The model under review builds one solid part; all positions refer to its coordinate system, in mm. Face numbers are marked on the shaded views. Coordinates: 2 decimals unless noted, no trailing zeros. Order: outer loops, then holes, each group sorted by start corner. A loop starts at its lowest first (then second) coordinate and runs counter-clockwise, first axis right, second up. Notation, with made-up numbers: (47, -4.75) -> (100, -4.75) arc R17 cw to (100, -0.75) -> close; hole circle Ø7 at (79.5, 16). An arc over 180 degrees is marked (long way). Put each result on its own line as item: value.
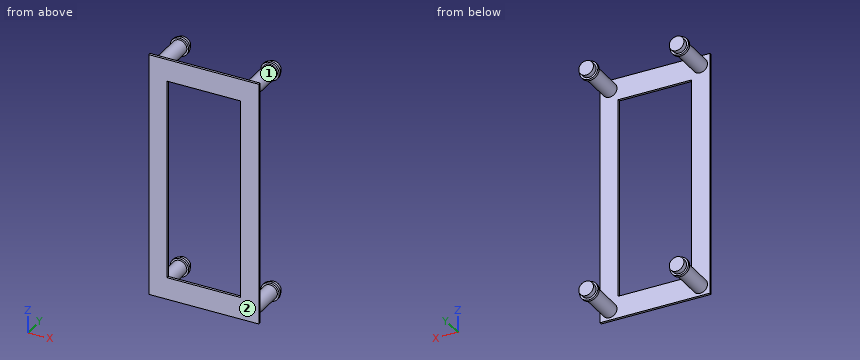
Autodesk Fusion 360 part; units mm, degrees
sketch "Sketch1" plane through (0, 0, 0) normal (0, 1, 0) x (1, 0, 0)
  line L0 (22.5, 50) -> (-22.5, 50)
  line L1 (-22.5, 50) -> (-22.5, -50)
  line L2 (-22.5, -50) -> (22.5, -50)
  line L3 (22.5, -50) -> (22.5, 50)
  line L4 (22.5, 50) -> (-22.5, -50) construction
  line L5 (-22.5, 50) -> (22.5, -50) construction
  line L6 (15, 41) -> (-15, 41)
  line L7 (-15, 41) -> (-15, -41)
  line L8 (-15, -41) -> (15, -41)
  line L9 (15, -41) -> (15, 41)
  line L10 (15, 41) -> (-15, -41) construction
  line L11 (-15, 41) -> (15, -41) construction
  dimension "d1" = 45
  dimension "d2" = 100
  dimension "d3" = 30
  dimension "d4" = 82
extrude "Extrude1" add sketch "Sketch1" along normal blind 1
sketch "Sketch2" plane through (0, 1, 0) normal (0, 1, 0) x (-1, 0, 0)
  line L0 (-15, -41) -> (-15, 41)
  line L1 (-15, 41) -> (15, 41)
  line L2 (15, 41) -> (15, -41)
  line L3 (15, -41) -> (-15, -41)
  line L4 (-22.5, 50) -> (-22.5, -50)
  line L5 (-22.5, -50) -> (22.5, -50)
  line L6 (22.5, -50) -> (22.5, 50)
  line L7 (22.5, 50) -> (-22.5, 50)
  circle A0 centre (18.5, -46) radius 3
  circle A1 centre (-18.5, -46) radius 3
  circle A2 centre (-18.5, 46) radius 3
  circle A3 centre (18.5, 46) radius 3
  dimension "d7" = 6
  dimension "d8" = 4
  dimension "d9" = 4
  dimension "d10" = 6
  dimension "d11" = 4
  dimension "d12" = 4
  dimension "d13" = 6
  dimension "d14" = 4
  dimension "d15" = 4
  dimension "d16" = 6
  dimension "d17" = 4
  dimension "d18" = 4
extrude "Extrude2" add sketch "Sketch2" along normal blind 15 contours A0 | A1 | A2 | A3
sketch "Sketch3" plane through (0, 16, 0) normal (0, 1, 0) x (-1, 0, 0)
  circle A0 centre (18.5, -46) radius 3
  circle A1 centre (18.5, -46) radius 3.75
  circle A2 centre (-18.5, -46) radius 3.75
  circle A3 centre (-18.5, -46) radius 3
  circle A4 centre (18.5, 46) radius 3.75
  circle A5 centre (18.5, 46) radius 3
  circle A6 centre (-18.5, 46) radius 3.75
  circle A7 centre (-18.5, 46) radius 3
  dimension "d21" = 7.5
  dimension "d22" = 7.5
  dimension "d23" = 7.5
  dimension "d24" = 7.5
extrude "Extrude3" add sketch "Sketch3" along normal blind 1 contours A0 | A1 | A2 | A3 | A4 | A5 | A6 | A7
sketch "Sketch4" plane through (0, 17, 0) normal (0, 1, 0) x (-1, 0, 0)
  circle A0 centre (-18.5, -46) radius 3.75
  circle A1 centre (-18.5, -46) radius 3
  circle A2 centre (18.5, -46) radius 3
  circle A3 centre (18.5, -46) radius 3.75
  circle A4 centre (-18.5, 46) radius 3
  circle A5 centre (-18.5, 46) radius 3.75
  circle A6 centre (18.5, 46) radius 3
  circle A7 centre (18.5, 46) radius 3.75
  dimension "d27" = 6
  dimension "d28" = 6
  dimension "d29" = 6
  dimension "d30" = 6
extrude "Extrude4" add sketch "Sketch4" along normal blind 2 contours A1 | A2 | A4 | A6
Item 1: For pin 1 Ø8 at (x, y) = (16, 2) entering from -Z; pin 2 Ø2 at (x, y) = (15.5, 8) entering from +Z; pin 3 Ø10 at (x, y) = (-16.5, 10) entering from -Z; pin 4 Ø10 at (x, y) = (-16, 16.5) entering from -Z, all flat-tipped, find the tip position at first contact; note any pin that passes through.
Answers below:
pin 1: z = -50
pin 2: z = 48.24
pin 3: z = -49
pin 4: z = -49.75
Item 2: For line 1 (Z direction, x = 18, y = 17.75); line 2 (Y direction, x = -14, z = 46), list the stretches that pass through material, from the lowest coordinate up. Write a range as from..to.
Answers below:
line 1: -48.96..-43.04, 43.04..48.96
line 2: 0..1
Item 3: Consider section C-C on y = 15. Write out the cut boundary in (x, z), and give its area (3 significant figures).
Answers below:
outline: circle Ø6 at (-18.5, -46); circle Ø6 at (-18.5, 46); circle Ø6 at (18.5, -46); circle Ø6 at (18.5, 46)
area: 113 mm^2
Item 4: Consider section A-A on z = 38. Write out the cut boundary in (x, y), and give its area (3 significant figures).
Answers below:
outline: (-22.5, 0) -> (-15, 0) -> (-15, 1) -> (-22.5, 1) -> close; (15, 0) -> (22.5, 0) -> (22.5, 1) -> (15, 1) -> close
area: 15.0 mm^2
Item 5: Consider section D-D on x = 18.5. Write out the cut boundary in (y, z), and give its area (3 significant figures).
Answers below:
outline: (0, -50) -> (1, -50) -> (1, -49) -> (16, -49) -> (16, -49.75) -> (17, -49.75) -> (17, -49) -> (19, -49) -> (19, -43) -> (17, -43) -> (17, -42.25) -> (16, -42.25) -> (16, -43) -> (1, -43) -> (1, 43) -> (16, 43) -> (16, 42.25) -> (17, 42.25) -> (17, 43) -> (19, 43) -> (19, 49) -> (17, 49) -> (17, 49.75) -> (16, 49.75) -> (16, 49) -> (1, 49) -> (1, 50) -> (0, 50) -> close
area: 319 mm^2
Item 6: Mouldability with a two-part tool opening along X and no side actions: class the marked faces 1 and 2 as +X half, -X half, draft (parallel to the pull), parting line (faces both ways), or undercut.
Answers below:
face 1: undercut
face 2: draft
Item 7: Consider section B-B on x = 6.5. Write out the cut boundary in (y, z).
Answers below:
outline: (0, -50) -> (1, -50) -> (1, -41) -> (0, -41) -> close; (0, 41) -> (1, 41) -> (1, 50) -> (0, 50) -> close
